Geometry: see drawing. Coordinates: mm, zero at the bounding-box minimum. A direction names the side the tool comes from. Coordinates: 2 decimals unless noted, no trailing zeros. Order: outer loops, then holes, each group sorted by start corner. A loop starts at its lowest first (then second) coordinate and runs counter-clockwise, first axis right, second up.
Item 1: Ray query, line 1 (Y direction, x = 3, z = 1.75); line 2 (X direction, y = 3, z = 1.25); line 3 (Y direction, x = 25, z = 3.6). Return the intervals inside material, ascending.
Item 2: Section A-A on z = 3.25. Return the cut outline in (x, y).
Item 3: Reachability of the marked faces 5, 6 and 7 from +Z, -Z, +X, -X, +Y, -Y: full face, straight path, thin tool, end or side. Return the list, or none.
Item 4: Section D-D on y = 3. Return the cut outline in (x, z).
Item 5: Section C-C on x = 22.25. Return the cut outline in (y, z).
Item 6: Contact query for a flat-ended pin moving along its axis: P1, Ø7.5, axis at x = 13, y = 11, coming from the +Z side. Output: stop coordinate, or through.
Item 7: Section B-B on y = 11. Return the cut outline in (x, z), then the cut area to 3 significant figures.
Item 8: Mould query, pull axis X, two halves, no side actions, for the marked faces 1, 2, 3 and 4. Classes: released by +X, released by -X, zero draft, split by the parting line, or undercut.
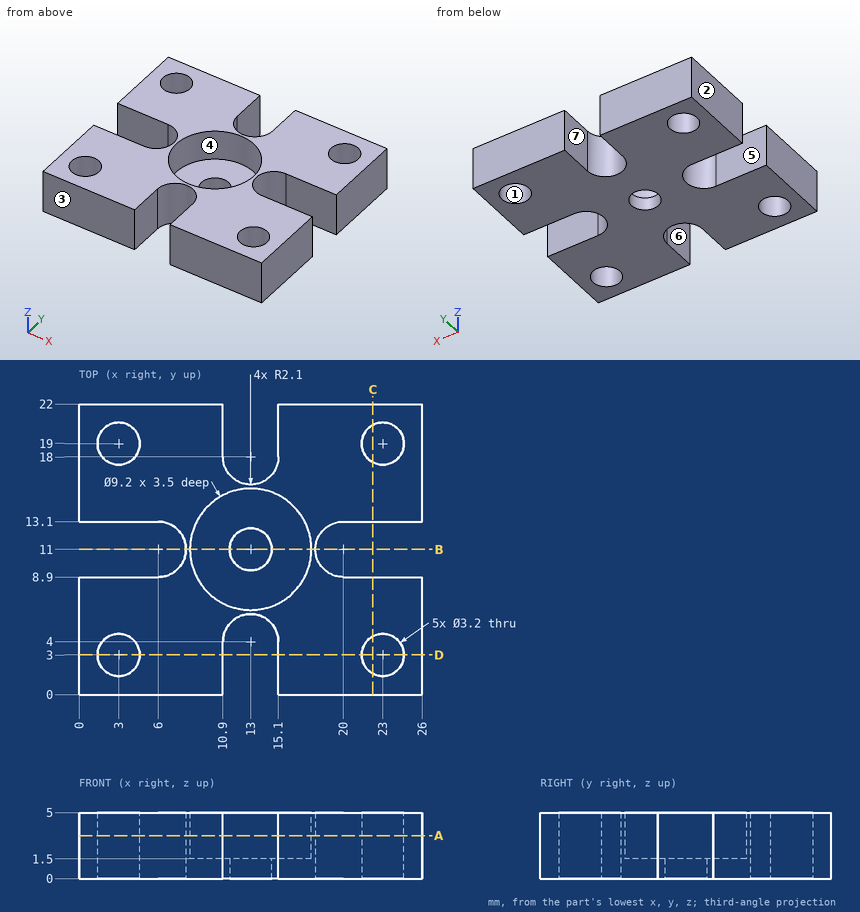
Answer list:
1. line 1: y = 0 to 1.4, 4.6 to 8.9, 13.1 to 17.4, 20.6 to 22
1. line 2: x = 0 to 1.4, 4.6 to 10.9, 15.1 to 21.4, 24.6 to 26
1. line 3: y = 0 to 8.9, 13.1 to 22
2. outline: (0, 0) - (10.9, 0) - (10.9, 4) arc R2.1 cw to (15.1, 4) - (15.1, 0) - (26, 0) - (26, 8.9) - (20, 8.9) arc R2.1 cw to (20, 13.1) - (26, 13.1) - (26, 22) - (15.1, 22) - (15.1, 18) arc R2.1 cw to (10.9, 18) - (10.9, 22) - (0, 22) - (0, 13.1) - (6, 13.1) arc R2.1 cw to (6, 8.9) - (0, 8.9) - close; hole circle Ø3.2 at (3, 3); hole circle Ø3.2 at (3, 19); hole circle Ø9.2 at (13, 11); hole circle Ø3.2 at (23, 3); hole circle Ø3.2 at (23, 19)
3. face 5: +Z, -Z, -X
3. face 6: +Z, -Z, -Y
3. face 7: +Z, -Z, +Y
4. outline: (0, 0) - (1.4, 0) - (1.4, 5) - (0, 5) - close; (4.6, 0) - (10.9, 0) - (10.9, 5) - (4.6, 5) - close; (15.1, 0) - (21.4, 0) - (21.4, 5) - (15.1, 5) - close; (24.6, 0) - (26, 0) - (26, 5) - (24.6, 5) - close
5. outline: (0, 0) - (1.59, 0) - (1.59, 5) - (0, 5) - close; (4.41, 0) - (8.9, 0) - (8.9, 5) - (4.41, 5) - close; (13.1, 0) - (17.59, 0) - (17.59, 5) - (13.1, 5) - close; (20.41, 0) - (22, 0) - (22, 5) - (20.41, 5) - close
6. P1: stops at z = 1.5
7. outline: (8.1, 0) - (11.4, 0) - (11.4, 1.5) - (8.4, 1.5) - (8.4, 5) - (8.1, 5) - close; (14.6, 0) - (17.9, 0) - (17.9, 5) - (17.6, 5) - (17.6, 1.5) - (14.6, 1.5) - close
7. area: 12.0 mm2
8. face 1: undercut
8. face 2: released by -X
8. face 3: zero draft
8. face 4: undercut
